Design review of the part built by this model. Coordinates are the model's own, in mm. Give positions to 0.01 mm unless a question says otherwise; leave off trailing zeros. Order: outer loops, then holes, each group sorted by start corner. A loop starts at its lowest first (then second) coordinate and runs counter-clockwise, first axis right, second up. Notation, with made-up numbers: (-27.75, 55.5) -> (-17.75, 55.5) arc R4 ccw to (-17.75, 60.5) -> close; hole circle Ø2 at (19, 19.25). An arc over 180 degrees is marked (long way). Use a Markdown table: item, result. Add a question column.
Solid Edge part; units mm, degrees
sketch "Sketch1" plane through (0, 0, -6.6) normal (0, 0, 1) x (1, 0, 0)
  line L0 (-40, -122.8657) -> (-40, -638.8657)
  line L1 (-33.5, -645.3657) -> (33.5, -645.3657)
  line L2 (40, -638.8657) -> (40, -122.8657)
  line L3 (33.5, -116.3657) -> (12.5, -116.3657)
  line L4 (6.5954, -154.6183) -> (6, -122.8657)
  line L5 (-6.5954, -154.6183) -> (-6.0046, -123.1094)
  line L6 (-12.5, -116.3657) -> (-33.5, -116.3657)
  arc A0 (-40, -638.8657) -> (-33.5, -645.3657) centre (-33.5, -638.8657) ccw
  arc A1 (33.5, -645.3657) -> (40, -638.8657) centre (33.5, -638.8657) ccw
  arc A2 (33.5, -116.3657) -> (40, -122.8657) centre (33.5, -122.8657) cw
  arc A3 (12.5, -116.3657) -> (6, -122.8657) centre (12.5, -122.8657) ccw
  arc A4 (6.5954, -154.6183) -> (-6.5954, -154.6183) centre (0, -154.8657) cw
  arc A5 (-12.5, -116.3657) -> (-6.0046, -123.1094) centre (-12.5, -122.8657) cw
  arc A6 (-33.5, -116.3657) -> (-40, -122.8657) centre (-33.5, -122.8657) ccw
  line L7 (-42, -122.8657) -> (-42, -638.8657)
  arc A7 (-42, -638.8657) -> (-33.5, -647.3657) centre (-33.5, -638.8657) ccw
  line L8 (-33.5, -647.3657) -> (33.5, -647.3657)
  arc A8 (33.5, -647.3657) -> (42, -638.8657) centre (33.5, -638.8657) ccw
  line L9 (42, -638.8657) -> (42, -122.8657)
  arc A9 (42, -122.8657) -> (33.5, -114.3657) centre (33.5, -122.8657) ccw
  line L10 (33.5, -114.3657) -> (12.5, -114.3657)
  arc A10 (12.5, -114.3657) -> (4, -122.8857) centre (12.5, -122.8657) ccw
  line L11 (4, -122.8857) -> (4.5961, -154.6762)
  arc A11 (4.5961, -154.6762) -> (-4.5961, -154.6762) centre (0, -154.8657) cw
  line L12 (-4.5961, -154.6762) -> (-4.0052, -123.1644)
  arc A12 (-4.0052, -123.1644) -> (-12.5, -114.3657) centre (-12.5, -122.8657) ccw
  line L13 (-12.5, -114.3657) -> (-33.5, -114.3657)
  arc A13 (-33.5, -114.3657) -> (-42, -122.8657) centre (-33.5, -122.8657) ccw
extrude "Protrusion1" add sketch "Sketch1" along normal blind 6
properties material "PVC"
1) Add section A-A (x = -21.5). Give the boundary of the cut face in (y, z).
2) Add section B-B (y = -384.5). Give the boundary of the cut face in (x, z), then the cut area to 3 significant figures.
3) Add section C-C (z = -5.15). Give the boundary of the cut face in (x, y).
4) The part is to be moulded in two halves that separate along X. For faces 1 (the cylindrical face through (39.444, -116.79, -3.642)), 2 (the cylindrical face through (-6.452, -116.893, -3.642)), 3 (the flat face through (40.2, -379.6, -6.6)), say which applies: +X half, -X half, draft (parallel to the pull), parting line (faces both ways), or undercut.
5) Insertion check: pin 1 (1.5 mm diameter, centred on x = 5.5, z = -2.5, fed in from +Y). The pin has a flat end and moves straight along its axis. Give the tip position at first contact, or say it passes through.
6) For L1, parallel to X at y = -152, z = -5.35; L2, parallel to X at y = -371.5, z = -1.05; L3, parallel to Y at x = -19, z = -5.5, list the stretches that pass through material, from the lowest coordinate up. Write a range as [from, to].
Worked answers:
| question | item | result |
|---|---|---|
| 1 | outline | (-647.37, -6.6) -> (-645.37, -6.6) -> (-645.37, -0.6) -> (-647.37, -0.6) -> close; (-116.37, -6.6) -> (-114.37, -6.6) -> (-114.37, -0.6) -> (-116.37, -0.6) -> close |
| 2 | outline | (-42, -6.6) -> (-40, -6.6) -> (-40, -0.6) -> (-42, -0.6) -> close; (40, -6.6) -> (42, -6.6) -> (42, -0.6) -> (40, -0.6) -> close |
| 2 | area | 24.0 mm^2 |
| 3 | outline | (-42, -638.87) arc R8.5 ccw to (-33.5, -647.37) -> (33.5, -647.37) arc R8.5 ccw to (42, -638.87) -> (42, -122.87) arc R8.5 ccw to (33.5, -114.37) -> (12.5, -114.37) arc R8.5 ccw to (4, -122.89) -> (4.6, -154.68) arc R4.6 cw (long way) to (-4.6, -154.68) -> (-4.01, -123.16) arc R8.5 ccw to (-12.5, -114.37) -> (-33.5, -114.37) arc R8.5 ccw to (-42, -122.87) -> close; hole (-40, -638.87) arc R6.5 ccw to (-33.5, -645.37) -> (33.5, -645.37) arc R6.5 ccw to (40, -638.87) -> (40, -122.87) arc R6.5 ccw to (33.5, -116.37) -> (12.5, -116.37) arc R6.5 ccw to (6, -122.87) -> (6.6, -154.62) arc R6.6 cw (long way) to (-6.6, -154.62) -> (-6, -123.11) arc R6.5 ccw to (-12.5, -116.37) -> (-33.5, -116.37) arc R6.5 ccw to (-40, -122.87) -> close |
| 4 | face 1 | +X half |
| 4 | face 2 | undercut |
| 4 | face 3 | draft |
| 5 | pin 1 | y = -117.1 |
| 6 | L1 | [-42, -40], [-6.55, -4.55], [4.55, 6.55], [40, 42] |
| 6 | L2 | [-42, -40], [40, 42] |
| 6 | L3 | [-647.37, -645.37], [-116.37, -114.37] |
